```python
from build123d import *

# Parameters (mm, degrees)
F0_R     = 11
F1_DEPTH = 3
F2_R     = 1.4
F3_DEPTH = 3


with BuildPart() as f1:
    # F0 (on Top) → F1 (new body)
    with BuildSketch(Plane.XY):
        Circle(F0_R)
        Polygon((4.7552825815, -1.5450849719), (0, -5), (-4.7552825815, -1.5450849719), (-2.9389262615, 4.0450849719), (2.9389262615, 4.0450849719), align=None, mode=Mode.SUBTRACT)
    extrude(amount=F1_DEPTH)

    # F2 (on face) → F3 (join)
    with BuildSketch(Plane.XY.offset(3)):
        with Locations((7.9, 0)):
            Circle(F2_R)
    extrude(amount=F3_DEPTH)

    # F4: F1 across plane


with BuildPart() as f1_1:
    add(f1.part)
    add(f1.part.mirror(Plane.YZ))


solid = f1_1.part
```
For this review, take the finished solid that the model builds, in its own axes (mm). A direction names the side the tool comes from. Round coordinates to 2 decimals unless told otherwise and drop trailing zeros. Write each loop counter-clockwise with the first axis right and the second up, starting at its lowest first coordinate (ties: lowest second). Pieces come first, ordered by that corner, then holes. Notation, with made-up numbers: (78, 78.25) -> (118, 78.25) arc R18 cw to (118, 104.25) -> close; hole circle Ø8 at (45, 63). An arc over 180 degrees is marked (long way). Use one line per item in the form item = value.
Q1. Consider section C-C (x = -3.75). State the section outline as (y, z) points, then the cut area to 3 significant figures.
Resolved:
outline = (-10.34, 0) -> (-2.28, 0) -> (-2.28, 3) -> (-10.34, 3) -> close; (1.55, 0) -> (10.34, 0) -> (10.34, 3) -> (1.55, 3) -> close
area = 50.6 mm²
Q2. The part is to be moulded in two halves that separate along Y. For faces 4 (the flat face through (-2.34, -3.3, 1.48)), 5 (the flat face through (0, 4.045, 1)), 6 (the flat face through (5, 0, 3)), 7 (the cylindrical face through (-6.5, 0.06, 4.48)), say which applies: released by +Y, released by -Y, zero draft, split by the parting line, or undercut.
Resolved:
face_4 = undercut
face_5 = undercut
face_6 = zero draft
face_7 = split by the parting line
Q3. Clearance check with flat-ended pins moving along their axes: pin 1 Ø2 at (x, z) = (7.5, 3.5) entering from -Y; pin 2 Ø1.5 at (x, z) = (-8.5, 4) entering from +Y; pin 3 Ø2 at (x, z) = (-4, 2) entering from +Y. State where each tip first meets the part, or that it passes through.
Resolved:
pin_1 = -8.77
pin_2 = 1.4
pin_3 = 10.58
Q4. To check wall thickness, follow probe 1 along Z at (x, y) = (1.25, -5); probe 2 along X at (y, z) = (2.25, 1); probe 3 along Y at (x, z) = (2.5, 2.05). State the ranges of each line that lie inside material, in increasing order. Write a range as from..to.
Resolved:
probe_1 = 0..3
probe_2 = -10.77..-3.52, 3.52..10.77
probe_3 = -10.71..-3.18, 4.05..10.71
Q5. Machinability: for faces 1 (the flat face through (5, 0, 0)), 2 (the cylindrical face through (6.5, 0.06, 4.48)), 3 (the flat face through (3.834, 1.289, 1.479)), which of the approach directions +Z, -Z, +X, -X, +Y, -Y give a long, thin tool a straight path to every point of the face, cutting with its end or side? Answer none if there is none.
Resolved:
face_1 = -Z, +X, -X, +Y, -Y
face_2 = +Z
face_3 = +Z, -Z
Q6. Consider section A-A (y = 3.5). State the section outline as (x, z) points.
Resolved:
outline = (-10.43, 0) -> (-3.12, 0) -> (-3.12, 3) -> (-10.43, 3) -> close; (3.12, 0) -> (10.43, 0) -> (10.43, 3) -> (3.12, 3) -> close
Q7. Consider section B-B (z = 1.85). State the section outline as (x, y) points, then the cut area to 3 significant figures.
Resolved:
outline = circle Ø22 at (0, 0); hole (-4.76, -1.55) -> (0, -5) -> (4.76, -1.55) -> (2.94, 4.05) -> (-2.94, 4.05) -> close
area = 321 mm²
Q8. Consider section D-D (z = 4.4). State the section outline as (x, y) points, then the cut area to 3 significant figures.
Resolved:
outline = circle Ø2.8 at (-7.9, 0); circle Ø2.8 at (7.9, 0)
area = 12.3 mm²
